Source: CAD feature listing. Evaluate the final solid. Frame: model axes, mm. A direction names the side the tool comes from. Coordinates: 2 decimals unless noted, no trailing zeros. Write each loop counter-clockwise with the first axis right and the second up, starting at its lowest first coordinate (ties: lowest second). Pieces come first, ordered by that corner, then holes. Notation, with made-up numbers: (3, 89.25) - (22, 89.25) arc R22 cw to (22, 105.25) - close; hole circle Ø7 at (-16.5, -28.75). An arc over 180 degrees is marked (long way). One line per question, with ' | ' between items. Start each with the question number.
Q1. Cut plane A-A, the plane y = -1631. Return loops of the section in (x, z).
Q2. Cut plane C-C, the plane z = 14.5. Return loops of the section in (x, y).
Q3. Draft query along Y for faces 1 (the face through (848, -1618.29, 23)), 2 (the face through (848, -1616.29, 23)), 3 (the face through (848, -1641, 48)), 4 (the face through (848, -1666.29, 23)). Return one class per face: +Y half, -Y half, draft (parallel to the pull), parting line (faces both ways), or undercut.
Q4. Line query: line 1 (Z direction, x = 186, y = -1624.5); line 2 (Z direction, x = 142.5, y = -1620); line 3 (Y direction, x = 1495.5, z = 14). Output: solid intervals per line, ascending.
Q5. Cut plane B-B, the plane x = 800.5. Return loops of the section in (y, z).
Q6. Access query for faces 5 (the face through (1675.841, -1641, 47)), 6 (the face through (848, -1641, 46)). Directions: +Z, -Z, +X, -X, +Y, -Y. A direction counts if a zero-diameter tool reaches every point of the face in a straight line with its end or side. Return the directions, or none.
```python
from build123d import *

# Parameters (mm, degrees)
F0_W      = 50
F0_H      = 50
F0_W_2    = 46
F0_H_2    = 46
F1_DEPTH  = 860
F2_R      = 2.5
F3_R      = 2.5
F8_DEPTH  = 820
F9_ANGLE  = 90
F10_ANGLE = 90


with BuildPart() as f1:
    # F0 (on Top) → F1 (new body)
    with BuildSketch(Plane.XY):
        with Locations((-29.1589260101, 36.7100374773)):
            Rectangle(F0_W, F0_H)
        with Locations((-29.1589260101, 36.7100374773)):
            Rectangle(F0_W_2, F0_H_2, mode=Mode.SUBTRACT)
    extrude(amount=F1_DEPTH)

    # F2
    f2_edges = [f1.edges().sort_by_distance(p)[0] for p in [
        (-4.158926, 61.710037, 430),
        (-54.158926, 61.710037, 430),
        (-4.158926, 11.710037, 430),
        (-54.158926, 11.710037, 430),
    ]]
    fillet(f2_edges, radius=F2_R)

    # F3
    f3_edges = [f1.edges().sort_by_distance(p)[0] for p in [
        (-6.158926, 59.710037, 430),
        (-52.158926, 59.710037, 430),
        (-52.158926, 13.710037, 430),
        (-6.158926, 13.710037, 430),
    ]]
    fillet(f3_edges, radius=F3_R)


with BuildPart() as f4_1:
    # F4: copy of F1
    add(f1.part)


with BuildPart() as f6_1:
    # F6: copy of F1
    add(f1.part)


with BuildPart() as f1_1:
    add(f1.part)

    # F8 (add, symmetric): a face of the model
    f8_faces = [f1_1.faces().sort_by_distance(p)[0] for p in [
        (-29.1589260101, 13.0029306961, 860),
    ]]
    extrude(f8_faces, amount=F8_DEPTH, both=True)


with BuildPart() as f1_2:
    # F9: moved
    add(f1_1.part.rotate(Axis((-29.1589260101, 13.7100374773, 0), (1, 0, 0)), F9_ANGLE))


with BuildPart() as f1_3:
    # F10: moved
    add(f1_2.part.rotate(Axis((-4.1589260101, -1666.2899625227, 23), (0, 0, -1)), F10_ANGLE))


solid = f1_3.part
```
Reply:
1) outline: (-4.16, -2) - (1675.84, -2) - (1675.84, 0) - (-4.16, 0) - close; (-4.16, 46) - (1675.84, 46) - (1675.84, 48) - (-4.16, 48) - close
2) outline: (-4.16, -1666.29) - (1675.84, -1666.29) - (1675.84, -1664.29) - (-4.16, -1664.29) - close; (-4.16, -1618.29) - (1675.84, -1618.29) - (1675.84, -1616.29) - (-4.16, -1616.29) - close
3) face 1: undercut | face 2: +Y half | face 3: draft | face 4: -Y half
4) line 1: z = -2 to 0, 46 to 48 | line 2: z = -2 to 0.13, 45.87 to 48 | line 3: y = -1666.29 to -1664.29, -1618.29 to -1616.29
5) outline: (-1666.29, 0.5) arc R2.5 ccw to (-1663.79, -2) - (-1618.79, -2) arc R2.5 ccw to (-1616.29, 0.5) - (-1616.29, 45.5) arc R2.5 ccw to (-1618.79, 48) - (-1663.79, 48) arc R2.5 ccw to (-1666.29, 45.5) - close; hole (-1664.29, 2.5) arc R2.5 ccw to (-1661.79, 0) - (-1620.79, 0) arc R2.5 ccw to (-1618.29, 2.5) - (-1618.29, 43.5) arc R2.5 ccw to (-1620.79, 46) - (-1661.79, 46) arc R2.5 ccw to (-1664.29, 43.5) - close
6) face 5: +Z, -Z, +X, +Y, -Y | face 6: +X, -X
